Check sheet for the drawn part. Datum: minimum x, y, z corner. Units: mm. A direction names the side the tool comes from. Give positions to 0.01 mm unless a question says otherwise; leave off trailing zeros. Order: outer loops, then holes, each group sorted by start corner. A loop starts at its lowest first (then second) coordinate and runs counter-clockwise, first axis right, second up.
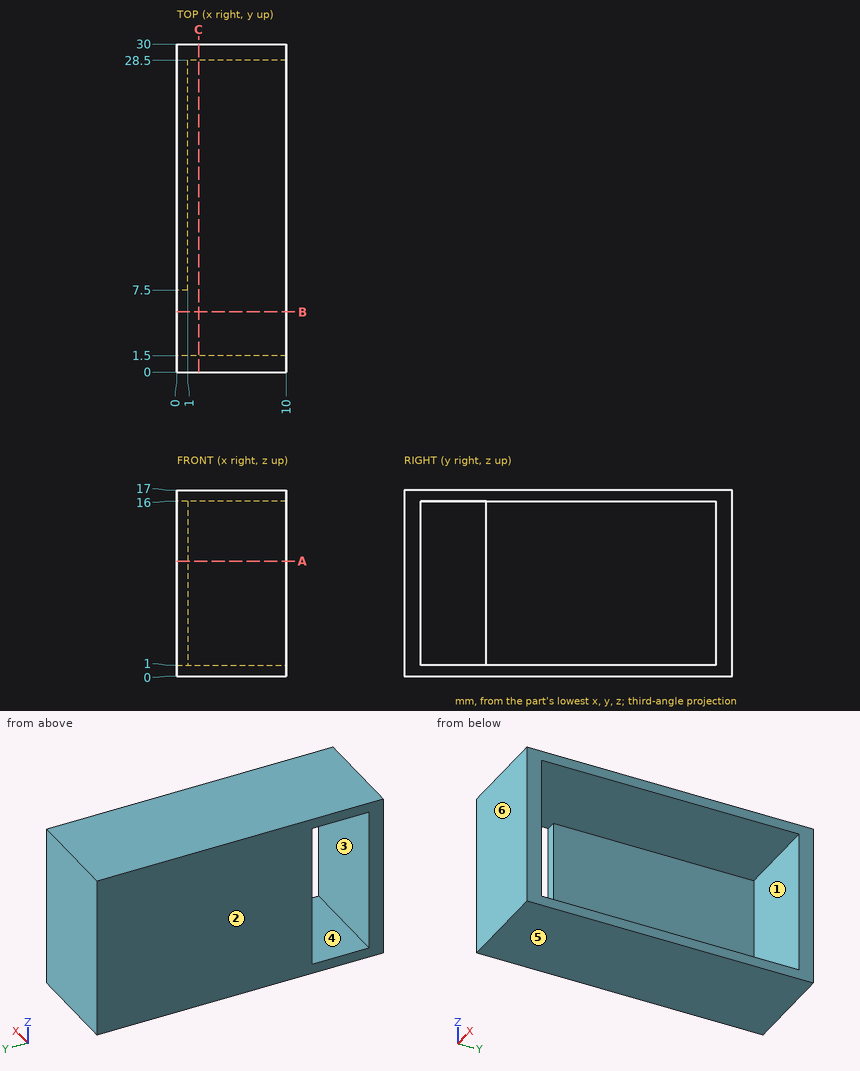
Item 1: Sectioned sample at B-B (y = 5.5). Enter the section's corners in (x, z), and give its area (3 significant figures).
Reported:
outline: (0, 0) - (10, 0) - (10, 1) - (0, 1) - close; (0, 16) - (10, 16) - (10, 17) - (0, 17) - close
area: 20.0 mm2
Item 2: Gauge pin test, flat end, axial feed: pin 1 (5 mm diameter, centred on y = 22.5, z = 9, fed in from +X). Record the tip position at first contact, or that the pin passes through.
Reported:
pin 1: stops at x = 1
Item 3: Sectioned sample at C-C (x = 2). Enter the section's corners in (y, z), and give its area (3 significant figures).
Reported:
outline: (0, 0) - (30, 0) - (30, 17) - (0, 17) - close; hole (1.5, 1) - (28.5, 1) - (28.5, 16) - (1.5, 16) - close
area: 105 mm2
Item 4: Draft check along Y on the marked faces 4, 5 and 6. Enter one of: released by +Y, released by -Y, zero draft, split by the parting line, or undercut.
Reported:
face 4: undercut
face 5: zero draft
face 6: released by -Y
Item 5: Set-up check for the marked faces 1, 2 and 3: record each of +Z, -Z, +X, -X, +Y, -Y from which the full face is reachable in a straight line by a thin tool's end or side.
Reported:
face 1: +X
face 2: +Z, -Z, -X, +Y, -Y
face 3: +X, -X
Item 6: Scan lines: L1, parallel to Z at x = 3.25, y = 26.25; L2, parallel to Y at x = 2.5, z = 13.25; L3, parallel to X at y = 26, z = 12.5. Record each from-to range of solid material in increasing order.
Reported:
L1: z = 0 to 1, 16 to 17
L2: y = 0 to 1.5, 28.5 to 30
L3: x = 0 to 1
Item 7: Sectioned sample at A-A (z = 10.5). Enter the section's corners in (x, y).
Reported:
outline: (0, 0) - (10, 0) - (10, 1.5) - (0, 1.5) - close; (0, 7.5) - (1, 7.5) - (1, 28.5) - (10, 28.5) - (10, 30) - (0, 30) - close
